Can you work these out from the drawing? Everything is in mm from the part's minimum corner. Round coordinates to 2 decimals unless told otherwise and drop trailing zeros. Loops run counter-clockwise (first coordinate to the right, second up) from the corner with the lowest first, then second, coordinate; pieces in that order, holes last. Notation, with made-up numbers: (82, -18.75) -> (140, -18.75) arc R23 ccw to (140, 19.25) -> close; hole circle Ø2 at (88, 14.5). An arc over 180 degrees is marked (long way). One line per item, written item: value.
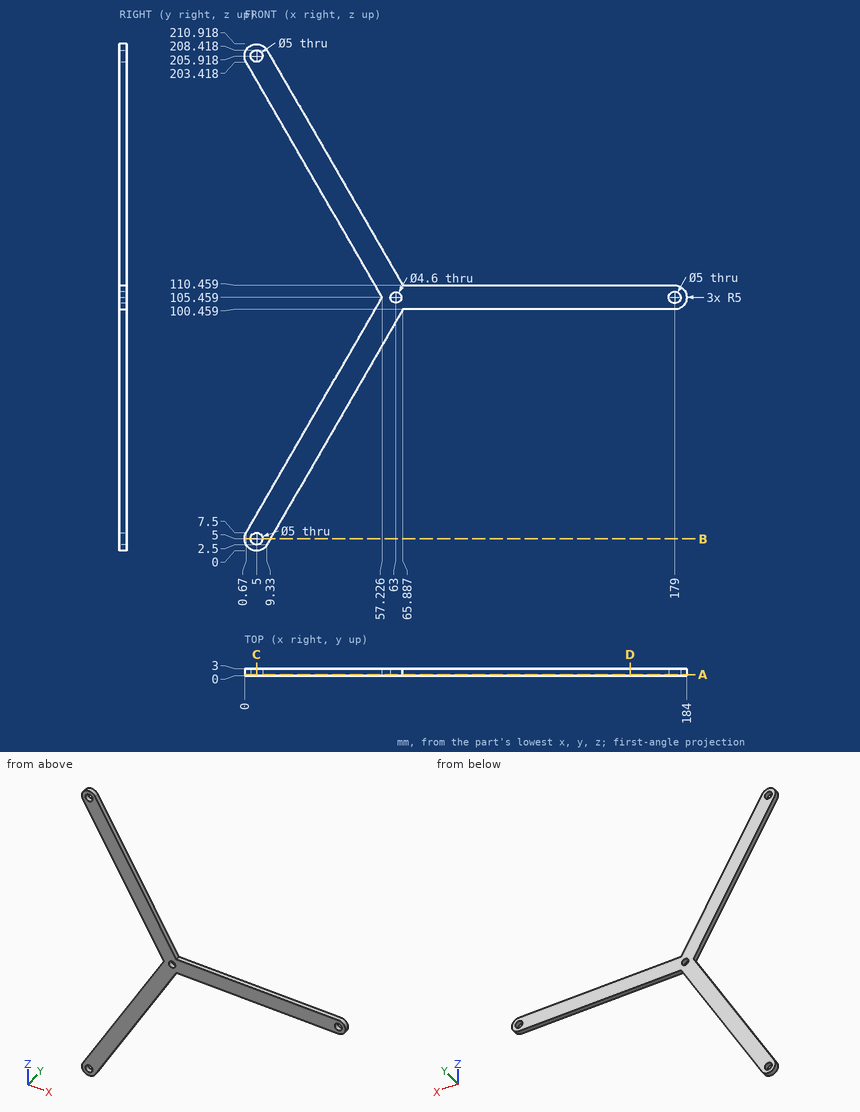
(1) If we section it at A-A, the plane y = 0.55: Please give me the cut outline in (x, z), then the cut area to 3 significant figures.
Recorded:
outline: (0.67, 7.5) arc R5 ccw to (9.33, 2.5) -> (65.89, 100.46) -> (179, 100.46) arc R5 ccw to (179, 110.46) -> (65.89, 110.46) -> (9.33, 208.42) arc R5 ccw to (0.67, 203.42) -> (57.23, 105.46) -> close; hole circle Ø5 at (5, 5); hole circle Ø5 at (5, 205.92); hole circle Ø4.6 at (63, 105.46); hole circle Ø5 at (179, 105.46)
area: 3,480 mm²
(2) If we section it at D-D, the plane x = 160.5: Please give me the cut outline in (y, z).
Recorded:
outline: (0, 100.46) -> (3, 100.46) -> (3, 110.46) -> (0, 110.46) -> close
(3) If we section it at C-C, the plane x = 5: Please give me the cut outline in (y, z).
Recorded:
outline: (0, 0) -> (3, 0) -> (3, 2.5) -> (0, 2.5) -> close; (0, 7.5) -> (3, 7.5) -> (3, 15) -> (0, 15) -> close; (0, 195.92) -> (3, 195.92) -> (3, 203.42) -> (0, 203.42) -> close; (0, 208.42) -> (3, 208.42) -> (3, 210.92) -> (0, 210.92) -> close
(4) If we section it at B-B, the plane z = 5: Please give me the cut outline in (x, y), then the cut area to 3 significant figures.
Recorded:
outline: (0, 0) -> (2.5, 0) -> (2.5, 3) -> (0, 3) -> close; (7.5, 0) -> (10.77, 0) -> (10.77, 3) -> (7.5, 3) -> close
area: 17.3 mm²
(5) I'm going to push flat-ended pins straight in: pin 1 Ø1 at (y, z) = (2.5, 44.5) entering from -X; pin 2 Ø3.5 at (x, z) = (63, 105.46) entering from +Y; pin 3 Ø1 at (y, z) = (2, 31.5) entering from -X; pin 4 Ø1.5 at (x, y) = (123.5, 1.5) entering from -Z. Where does each tip first touch, or does it pass through?
Recorded:
pin 1: x = 21.74
pin 2: through
pin 3: x = 14.24
pin 4: z = 100.46
(6) If I drill on L1, parallel to Z at x = 112.5, y = 1.45; L2, parallel to X at y = 1.7, z = 5 (1 decimal); L3, parallel to Z at x = 38, y = 1.95 (1 decimal), over which ranges is the centre line in solid material (lowest first)?
Recorded:
L1: 100.46 to 110.46
L2: 0 to 2.5, 7.5 to 10.8
L3: 52.2 to 72.2, 138.8 to 158.8
